from build123d import *

# Parameters (mm, degrees)
SKETCH1_W                      = 294
SKETCH1_H                      = 2402
BASE_FLANGE1_DEPTH             = 4
EDGE_FLANGE1_STRIP_W           = 28
EDGE_FLANGE1_STRIP_H           = 4
EDGE_FLANGE1_STRIP_CUT_DEPTH   = 2402
EDGE_FLANGE1_STRIP_2_W         = 28
EDGE_FLANGE1_STRIP_2_H         = 4
EDGE_FLANGE1_STRIP_CUT_2_DEPTH = 2402
EDGE_FLANGE1_DEPTH             = 2402
EDGE_FLANGE1_BEND_DEPTH        = 2402
SKETCH20_R                     = 8
CUT_EXTRUDE3_DEPTH             = 10
LPATTERN1_COUNT                = 2
LPATTERN1_PITCH                = 220
LPATTERN1_COUNT_DIR2           = 2
LPATTERN1_PITCH_DIR2           = 146
SKETCH21_R                     = 6
CUT_EXTRUDE4_DEPTH             = 10
SKETCH22_R                     = 6
CUT_EXTRUDE5_DEPTH             = 10
SKETCH23_R                     = 6
CUT_EXTRUDE6_DEPTH             = 1239.794979002


# Sheet-metal steps are written as plain solids
with BuildPart() as part:
    # Sketch1 → Base-Flange1 (new body)
    with BuildSketch(Plane(origin=(0, 0, 0), x_dir=(1, 0, 0), z_dir=(0, 1, 0))):
        Rectangle(SKETCH1_W, SKETCH1_H)
    extrude(amount=-BASE_FLANGE1_DEPTH)

    # Edge-Flange1 strip (across the edge) → Edge-Flange1 strip cut (cut)
    with BuildSketch(Plane(origin=(147, 0, 1201), x_dir=(-1, 0, 0), z_dir=(0, 0, -1))):
        with Locations((-4, -2)):
            Rectangle(EDGE_FLANGE1_STRIP_W, EDGE_FLANGE1_STRIP_H)
    extrude(amount=EDGE_FLANGE1_STRIP_CUT_DEPTH, mode=Mode.SUBTRACT)

    # Edge-Flange1 strip 2 (across the edge) → Edge-Flange1 strip cut 2 (cut)
    with BuildSketch(Plane(origin=(-147, 0, -1201), x_dir=(1, 0, 0), z_dir=(0, 0, 1))):
        with Locations((-4, -2)):
            Rectangle(EDGE_FLANGE1_STRIP_2_W, EDGE_FLANGE1_STRIP_2_H)
    extrude(amount=EDGE_FLANGE1_STRIP_CUT_2_DEPTH, mode=Mode.SUBTRACT)

    # Edge-Flange1 section (across the edge) → Edge-Flange1 (add)
    with BuildSketch(Plane(origin=(147, 0, 1201), x_dir=(-1, 0, 0), z_dir=(0, 0, -1))):
        with BuildLine():
            Line((0, 6), (0, 76))
            Line((0, 76), (4, 76))
            Line((4, 76), (4, 6))
            ThreePointArc((4, 6), (5.757359313, 1.757359313), (10, 0))
            Line((10, 0), (10, -4))
            ThreePointArc((10, -4), (2.928932188, -1.071067812), (0, 6))
        make_face()
    extrude(amount=EDGE_FLANGE1_DEPTH)

    # Edge-Flange1 section 2 (across the edge) → Edge-Flange1 bend (add)
    with BuildSketch(Plane(origin=(-147, 0, -1201), x_dir=(1, 0, 0), z_dir=(0, 0, 1))):
        with BuildLine():
            Line((0, 6), (0, 76))
            Line((0, 76), (4, 76))
            Line((4, 76), (4, 6))
            ThreePointArc((4, 6), (5.757359313, 1.757359313), (10, 0))
            Line((10, 0), (10, -4))
            ThreePointArc((10, -4), (2.928932188, -1.071067812), (0, 6))
        make_face()
    extrude(amount=EDGE_FLANGE1_BEND_DEPTH)

    # Sketch20 → Cut-Extrude3 (cut)
    with BuildSketch(Plane.XZ.offset(4)):
        with Locations(Location((-110, 73, 0), (0, 0, 270))):
            Circle(SKETCH20_R)
    cut_extrude3 = extrude(amount=-CUT_EXTRUDE3_DEPTH, mode=Mode.SUBTRACT)

    # LPattern1: Cut-Extrude3 2 × 2
    with Locations(*[(i * LPATTERN1_PITCH, 0, -j * LPATTERN1_PITCH_DIR2) for i in range(LPATTERN1_COUNT) for j in range(LPATTERN1_COUNT_DIR2) if (i, j) != (0, 0)]):
        add(cut_extrude3, mode=Mode.SUBTRACT)

    # Sketch21 → Cut-Extrude4 (cut)
    with BuildSketch(Plane.XZ.offset(4)):
        with Locations(Location((-122, 1156, 0), (0, 0, 270))):
            Circle(SKETCH21_R)
        with Locations(Location((122, 1156, 0), (0, 0, 270))):
            Circle(SKETCH21_R)
    cut_extrude4 = extrude(amount=-CUT_EXTRUDE4_DEPTH, mode=Mode.SUBTRACT)

    # Sketch22 → Cut-Extrude5 (cut)
    with BuildSketch(Plane.XZ.offset(4)):
        with Locations(Location((0, 1156, 0), (0, 0, 270))):
            Circle(SKETCH22_R)
    cut_extrude5 = extrude(amount=-CUT_EXTRUDE5_DEPTH, mode=Mode.SUBTRACT)

    # Sketch23 → Cut-Extrude6 (cut, through all)
    with BuildSketch(Plane.ZY.offset(147)):
        with Locations(Location((1176, 36, 0), (0, 0, 270))):
            Circle(SKETCH23_R)
    cut_extrude6 = extrude(amount=-CUT_EXTRUDE6_DEPTH, mode=Mode.SUBTRACT)

    # Mirror1: Cut-Extrude4, Cut-Extrude5, Cut-Extrude6 across plane
    add(cut_extrude4.mirror(Plane.XY), mode=Mode.SUBTRACT)
    add(cut_extrude5.mirror(Plane.XY), mode=Mode.SUBTRACT)
    add(cut_extrude6.mirror(Plane.XY), mode=Mode.SUBTRACT)


solid = part.part
Check sheet for the modelled part. Datum: model origin and axes. Units: mm. A direction names the side the tool comes from. Round coordinates to 2 decimals unless told otherwise and drop trailing zeros. Order: outer loops, then holes, each group sorted by start corner. A loop starts at its lowest first (then second) coordinate and runs counter-clockwise, first axis right, second up.
(1) Scan lines: probe 1 along X at (y, z) = (66, -210.5); probe 2 along X at (y, z) = (-2.6, 73); probe 3 along Y at (x, z) = (37, -869.5). Record each from-to range of solid material in increasing order.
(2) Cross-section at B-B, the plane x = 80. Enter the section's corners in (y, z).
(3) Go/stop test with flat-tipped pins: P1, Ø15.5, axis at x = 122, z = 1156, coming from the +Y side; P2, Ø18.5, axis at x = 110, z = 73, coming from the -Y side. Record where each tip stops, or that it passes through.
(4) Access from +Z, -Z, +X, -X, +Y, -Y to the whole of each face (thin tool, end or side, straight path). Record for faces 1 (the flat face through (-143, 41, -17)), 2 (the flat face through (-2, -4, -17)).
(5) Draft check along X on faces 3 (the flat face through (-2, 0, -17)), 4 (the flat face through (1, -2, 1201)), 5 (the flat face through (147, 41, 17)). Enter one of: pulls with the +X half, pulls with the -X half, needs draft (parallel to the pull), parting line crosses it, or undercut.
(6) Cross-section at A-A, the plane z = 366.5. Enter the section's corners in (x, y), and give its area (3 significant figures).
Check sheet entries:
1. probe 1: x = -147 to -143, 143 to 147
1. probe 2: x = -142.1 to -118, -102 to 102, 118 to 142.1
1. probe 3: y = -4 to 0
2. outline: (-4, -1201) - (0, -1201) - (0, 1201) - (-4, 1201) - close
3. P1: stops at y = 0
3. P2: stops at y = -4
4. face 1: +Z, -Z, +Y
4. face 2: +Z, -Z, +X, -X, -Y
5. face 3: undercut
5. face 4: needs draft
5. face 5: pulls with the +X half
6. outline: (-147, 6) arc R10 ccw to (-137, -4) - (137, -4) arc R10 ccw to (147, 6) - (147, 76) - (143, 76) - (143, 6) arc R6 cw to (137, 0) - (-137, 0) arc R6 cw to (-143, 6) - (-143, 76) - (-147, 76) - close
6. area: 1,760 mm2
